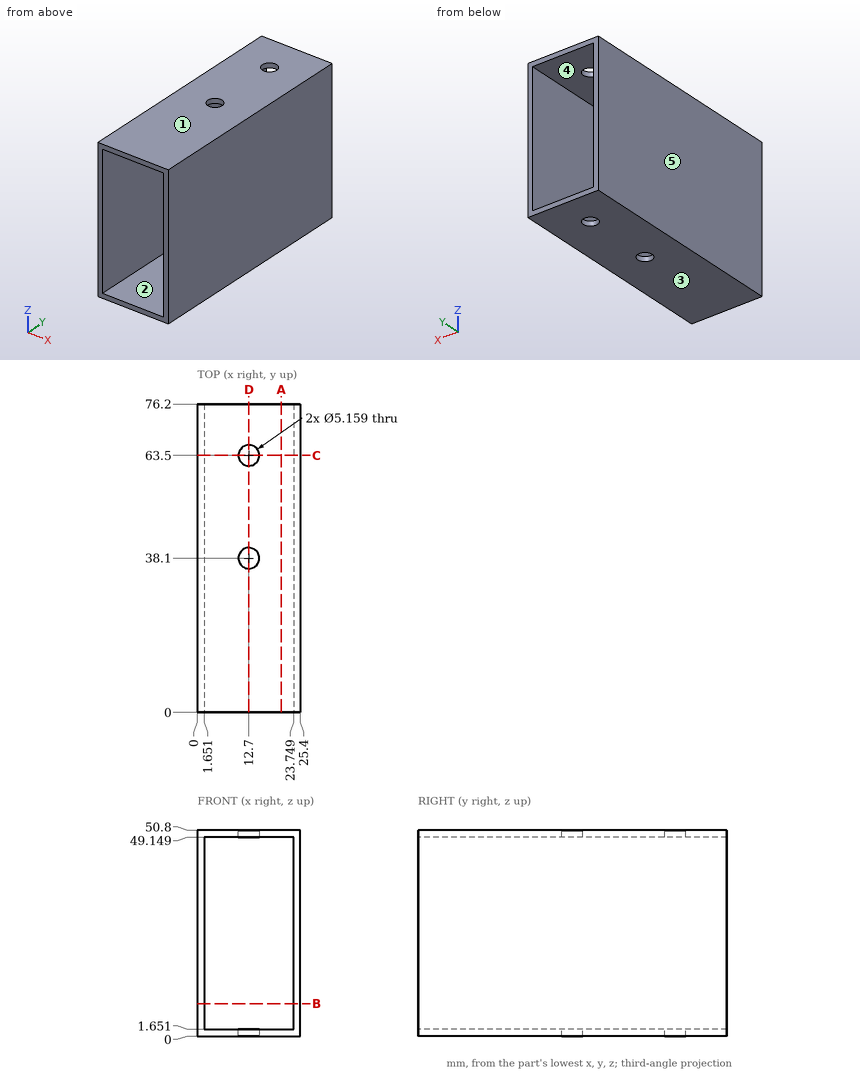
Geometry check sheet. Reference: drawing and pictorial views, mm from the part's lowest x, y, z. A direction names the side the tool comes from. Round coordinates to 2 decimals unless told otherwise and drop trailing zeros. Order: outer loops, then holes, each group sorted by start corner. A loop starts at its lowest first (then second) coordinate and runs counter-clockwise, first axis right, second up. Notation, with made-up numbers: M 32,65.25 L 55,65.25 A24 ccw 55,103.25 Z; hole C 41,20 d7. An arc over 180 degrees is marked long. Write item = value, one per line.
Q1. Scan lines: line 1 (X direction, y = 12.5, z = 26.5); line 2 (Z direction, x = 19.5, y = 14); line 3 (Y direction, x = 12.7, z = 0.8). Record each from-to range of solid material in increasing order.
Answer block:
line_1 = 0 to 1.65, 23.75 to 25.4
line_2 = 0 to 1.65, 49.15 to 50.8
line_3 = 0 to 35.52, 40.68 to 60.92, 66.08 to 76.2
Q2. Section check B-B (z = 8). Enter the section's corners in (x, y).
Answer block:
outline = M 0,0 L 1.65,0 L 1.65,76.2 L 0,76.2 Z; M 23.75,0 L 25.4,0 L 25.4,76.2 L 23.75,76.2 Z
Q3. Depth check by flat-ended pin: pin 1 Ø1.5 at (y, z) = (14, 13.5) entering from -X. Enter the tip coordinate at first touch or a pass-through.
Answer block:
pin_1 = 0
Q4. Release check for a two-part mould opening along Z. For the marked faces 3, 4 and 5 record: released by +Z, released by -Z, zero draft, split by the parting line, or undercut.
Answer block:
face_3 = released by -Z
face_4 = undercut
face_5 = zero draft
Q5. Section check A-A (x = 20.75). Enter the section's corners in (y, z).
Answer block:
outline = M 0,0 L 76.2,0 L 76.2,1.65 L 0,1.65 Z; M 0,49.15 L 76.2,49.15 L 76.2,50.8 L 0,50.8 Z
Q6. Set-up check for the marked faces 1 and 2: record each of +Z, -Z, +X, -X, +Y, -Y from which the full face is reachable in a straight line by a thin tool's end or side.
Answer block:
face_1 = +Z, +X, -X, +Y, -Y
face_2 = +Y, -Y
Q7. Section check D-D (x = 12.7). Enter the section's corners in (y, z).
Answer block:
outline = M 0,0 L 35.52,0 L 35.52,1.65 L 0,1.65 Z; M 0,49.15 L 35.52,49.15 L 35.52,50.8 L 0,50.8 Z; M 40.68,0 L 60.92,0 L 60.92,1.65 L 40.68,1.65 Z; M 40.68,49.15 L 60.92,49.15 L 60.92,50.8 L 40.68,50.8 Z; M 66.08,0 L 76.2,0 L 76.2,1.65 L 66.08,1.65 Z; M 66.08,49.15 L 76.2,49.15 L 76.2,50.8 L 66.08,50.8 Z
Q8. Section check C-C (y = 63.5). Enter the section's corners in (x, z).
Answer block:
outline = M 0,0 L 10.12,0 L 10.12,1.65 L 1.65,1.65 L 1.65,49.15 L 10.12,49.15 L 10.12,50.8 L 0,50.8 Z; M 15.28,0 L 25.4,0 L 25.4,50.8 L 15.28,50.8 L 15.28,49.15 L 23.75,49.15 L 23.75,1.65 L 15.28,1.65 Z
